Verification items for this drawing (mm, ordinates from the low corner). A direction names the side the tool comes from. Coordinates: 2 decimals unless noted, no trailing zeros. Order: outer loops, then holes, each group sorted by start corner. A loop starts at its lowest first (then second) coordinate and runs counter-clockwise, first axis right, second up. Notation, with made-up numbers: M 64,-39 L 83,-39 A22 ccw 83,-19 Z; hole C 50,-21.5 d3. An arc over 180 degrees is marked long. Answer as a JSON object with one key per item and string values. Group by question number.
(1) Gauge pin test, flat ends, axial feed: pin 1 Ø2.5 at (x, z) = (32, 18) entering from -Y; pin 2 Ø1 at (x, y) = (5.5, 10.5) entering from -Z; pin 3 Ø3.5 at (y, z) = (18.5, 4.5) entering from +X; pin 4 Ø6.5 at (x, y) = (36, 5) entering from +Z. Record the tip position at first contact, or that the pin passes through.
(2) Cross-section at B-B (x = 36). Enter the section's corners in (y, z).
(3) Cross-section at C-C (x = 20). Enter the section's corners in (y, z), plus the area to 3 significant figures.
(4) Cross-section at D-D (y = 9.25). Enter the section's corners in (x, z), plus the area to 3 significant figures.
(5) Access from +Z, -Z, +X, -X, +Y, -Y to the whole of each face (thin tool, end or side, straight path). Record for the marked faces 1 and 2.
(6) Material ranges on line 1 (Y direction, x = 4, z = 13); line 2 (X direction, y = 23, z = 24.25) (1 decimal); line 3 (X direction, y = 22, z = 22.5), recorded low to high.
(7) Cross-section at A-A (y = 5). Enter the section's corners in (x, z).
(8) Mould release check, pull along X, two halves, no side actions. Record for the marked faces 3, 4 and 5: released by +X, released by -X, zero draft, split by the parting line, or undercut.
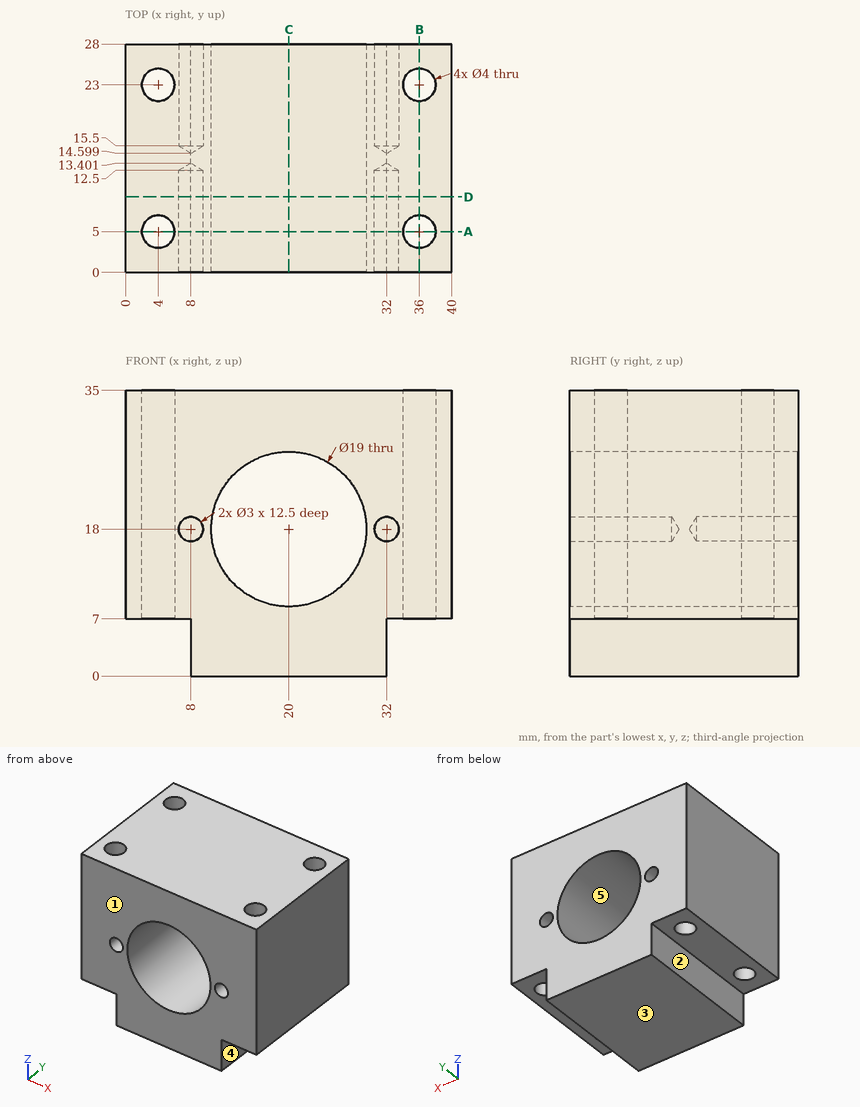
Taken from the geometry:
{
 "1": {"pin 1": "stops at y = 12.65", "pin 2": "stops at z = 7", "pin 3": "stops at x = 32", "pin 4": "stops at z = 35"},
 "2": {"outline": "M 0,7 L 3,7 L 3,35 L 0,35 Z; M 7,7 L 21,7 L 21,35 L 7,35 Z; M 25,7 L 28,7 L 28,35 L 25,35 Z"},
 "3": {"outline": "M 0,0 L 28,0 L 28,8.5 L 0,8.5 Z; M 0,27.5 L 28,27.5 L 28,35 L 0,35 Z", "area": "448 mm²"},
 "4": {"outline": "M 0,7 L 8,7 L 8,0 L 32,0 L 32,7 L 40,7 L 40,35 L 0,35 Z; hole C 8,18 d3; hole C 20,18 d19; hole C 32,18 d3", "area": "990 mm²"},
 "5": {"face 1": "+Z, -Z, +X, -X, -Y", "face 2": "-Z, -X, +Y, -Y"},
 "6": {"line 1": "y = 0 to 3, 7 to 21, 25 to 28", "line 2": "x = 0 to 2, 6 to 12.8, 27.2 to 34, 38 to 40", "line 3": "x = 0 to 2.27, 5.73 to 11.63, 28.37 to 34.27, 37.73 to 40"},
 "7": {"outline": "M 0,7 L 2,7 L 2,35 L 0,35 Z; M 6,7 L 8,7 L 8,0 L 32,0 L 32,7 L 34,7 L 34,35 L 6,35 Z; M 38,7 L 40,7 L 40,35 L 38,35 Z; hole C 8,18 d3; hole C 20,18 d19; hole C 32,18 d3"},
 "8": {"face 3": "zero draft", "face 4": "released by +X", "face 5": "undercut"}
}
